from build123d import *

# Parameters (mm, degrees)
F1_DEPTH = 3.175
F3_DEPTH = 3.175
F4_W     = 38.1
F4_H     = 15.875
F5_DEPTH = 1.5875
F7_W     = 95.25
F7_H     = 15.875
F8_DEPTH = 3.175
F9_R     = 12.7
F11_D    = 6.35
F12_R    = 3.175
F13_R    = 1.5875


with BuildPart() as f1:
    # F0 (on Front) → F1 (new body)
    with BuildSketch(Plane.XZ):
        Polygon((-47.625, 0), (0, 0), (47.625, 0), (47.625, 101.6), (0, 101.6), (-47.625, 101.6), align=None)
    extrude(amount=F1_DEPTH)

    # F2 (on Top) → F3 (join)
    with BuildSketch(Plane.XY):
        Polygon((47.625, 0), (0, 0), (-47.625, 0), (-47.625, -38.1), (0, -38.1), (47.625, -38.1), align=None)
    extrude(amount=F3_DEPTH)

    # F4 (on face) → F5 (join)
    with BuildSketch(Plane.YZ.offset(47.625)):
        with Locations((-19.05, 7.9375)):
            Rectangle(F4_W, F4_H)
    extrude(amount=-F5_DEPTH)

    # F6: F1 across plane


with BuildPart() as f1_1:
    add(f1.part)
    add(f1.part.mirror(Plane.YZ))

    # F7 (on face) → F8 (join)
    with BuildSketch(Plane.XZ.offset(38.1)):
        with Locations((0, 7.9375)):
            Rectangle(F7_W, F7_H)
    extrude(amount=F8_DEPTH)

    # F9
    f9_edges = [f1_1.edges().sort_by_distance(p)[0] for p in [
        (47.625, -1.5875, 101.6),
        (-47.625, -1.5875, 101.6),
    ]]
    fillet(f9_edges, radius=F9_R)

    # F11 (through all)
    with Locations(Plane.XZ.offset(3.175)):
        with Locations((0, 76.2)):
            Hole(F11_D / 2)

    # F12
    f12_edges = [f1_1.edges().sort_by_distance(p)[0] for p in [
        (-46.83125, -3.175, 15.875),
        (46.83125, -3.175, 15.875),
    ]]
    fillet(f12_edges, radius=F12_R)

    # F13
    f13_edges = [f1_1.edges().sort_by_distance(p)[0] for p in [
        (-47.625, -41.275, 7.9375),
        (47.625, -41.275, 7.9375),
    ]]
    fillet(f13_edges, radius=F13_R)


solid = f1_1.part
Verification items for the finished model (mm, model axes). A direction names the side the tool comes from. Coordinates: 2 decimals unless noted, no trailing zeros. Order: outer loops, then holes, each group sorted by start corner. A loop starts at its lowest first (then second) coordinate and runs counter-clockwise, first axis right, second up. Notation, with made-up numbers: (18, -5) -> (72, -5) arc R10 cw to (72, 0) -> close; hole circle Ø3 at (3, 3). An arc over 180 degrees is marked (long way). Put each result on its own line as item: value. Start each with the question number.
1. Access from +Z, -Z, +X, -X, +Y, -Y to the whole of each face (thin tool, end or side, straight path). Record for faces 1 (the flat face through (46.038, -21, 9)), 2 (the flat face through (-1, -20, 0)), 3 (the flat face through (-14, -39, 15.875)).
2. Go/stop test with flat-tipped pins: pin 1 Ø10 at (x, z) = (0, 76.2) entering from -Y (3 decimals); pin 2 Ø1 at (x, y) = (-1, -26.5) entering from +Z (3 decimals). Record where each tip stops, or that it passes through.
3. Material ranges on L1, parallel to X at y = -1, z = 76 (3 decimals); L2, parallel to Z at x = 0, y = -1.6 (3 decimals); L3, parallel to X at y = -37.5, z = 14.5 (1 decimal), recorded low to high. Write a range as [from, to].
4. Cross-section at D-D, the plane y = -12.5. Record the boundary of the cut face in (x, z) (1 decimal).
5. Mould release check, pull along Y, two halves, no side actions. Record for faces 4 (the flat face through (-1, -38.1, 10)), 5 (the flat face through (-1, 0, 52)), 6 (the flat face through (47.625, -15, 15)), 7 (the flat face through (-46.038, -21, 9)): released by +Y, released by -Y, zero draft, split by the parting line, or undercut.
6. Cross-section at A-A, the plane z = 76.2. Record the boundary of the cut face in (x, y) (3 decimals), then the cut area to 3 significant figures.
7. Cross-section at B-B, the plane x = 0. Record the boundary of the cut face in (y, z) (3 decimals).
8. Cross-section at C-C, the plane x = 11. Record the boundary of the cut face in (y, z) (3 decimals), then the cut area to 3 significant figures.
Computed:
1. face 1: +Z
1. face 2: -Z, +X, -X, +Y, -Y
1. face 3: +Z, +X, -X, -Y
2. pin 1: y = -3.175
2. pin 2: z = 3.175
3. L1: [-47.625, -3.169], [3.169, 47.625]
3. L2: [0, 73.025], [79.375, 101.6]
3. L3: [-47.6, -46], [46, 47.6]
4. outline: (-47.6, 0) -> (47.6, 0) -> (47.6, 15.9) -> (46, 15.9) -> (46, 3.2) -> (-46, 3.2) -> (-46, 15.9) -> (-47.6, 15.9) -> close
5. face 4: undercut
5. face 5: released by +Y
5. face 6: zero draft
5. face 7: undercut
6. outline: (-47.625, -3.175) -> (-3.175, -3.175) -> (-3.175, 0) -> (-47.625, 0) -> close; (3.175, -3.175) -> (47.625, -3.175) -> (47.625, 0) -> (3.175, 0) -> close
6. area: 282 mm2
7. outline: (-41.275, 0) -> (0, 0) -> (0, 73.025) -> (-3.175, 73.025) -> (-3.175, 3.175) -> (-38.1, 3.175) -> (-38.1, 15.875) -> (-41.275, 15.875) -> close; (-3.175, 79.375) -> (0, 79.375) -> (0, 101.6) -> (-3.175, 101.6) -> close
8. outline: (-41.275, 0) -> (0, 0) -> (0, 101.6) -> (-3.175, 101.6) -> (-3.175, 3.175) -> (-38.1, 3.175) -> (-38.1, 15.875) -> (-41.275, 15.875) -> close
8. area: 484 mm2
